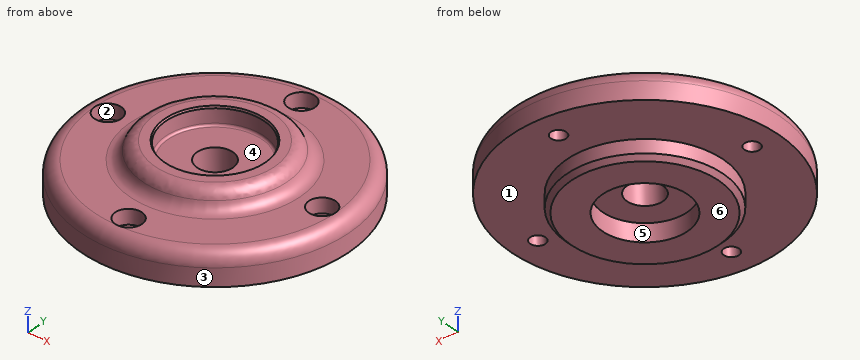
Autodesk Inventor part; units mm, degrees
ref_plane "YZ Plane" through (0, 0, 0) normal (1, 0, 0) x (0, 1, 0)
ref_plane "XZ Plane" through (0, 0, 0) normal (0, 1, 0) x (-1, 0, 0)
ref_plane "XY Plane" through (0, 0, 0) normal (0, 0, 1) x (1, 0, 0)
sketch "스케치4" plane through (0, 0, 0) normal (0, 0, 1) x (1, 0, 0)
  circle A0 centre (0, 0) radius 30
  dimension "d28" = 60
extrude "돌출4" add sketch "스케치4" along normal blind 7
sketch "스케치5" plane through (0, 0, 7) normal (0, 0, 1) x (1, 0, 0)
  circle A0 centre (0, 0) radius 16
  dimension "d31" = 32
extrude "돌출5" add sketch "스케치5" along normal blind 4
sketch "스케치6" plane through (0, 0, 0) normal (0, 0, -1) x (-1, 0, 0)
  circle A0 centre (0, 0) radius 17.5
  dimension "d34" = 35
extrude "돌출6" add sketch "스케치6" along normal blind 4
sketch "스케치8" plane through (0, 0, 11) normal (0, 0, 1) x (1, 0, 0)
  circle A0 centre (0, 0) radius 11
  dimension "d41" = 22
extrude "돌출8" cut sketch "스케치8" against normal blind 4
sketch "스케치9" plane through (0, 0, -4) normal (0, 0, -1) x (-1, 0, 0)
  circle A0 centre (0, 0) radius 9.5
  dimension "d44" = 19
extrude "돌출9" cut sketch "스케치9" against normal blind 4
sketch "스케치11" plane through (0, 0, 7) normal (0, 0, 1) x (1, 0, 0)
  circle A0 centre (0, 0) radius 4
  dimension "d49" = 8
extrude "돌출10" cut sketch "스케치11" against normal up to next
sketch "스케치12" plane through (0, 0, 7) normal (0, 0, 1) x (1, 0, 0)
  circle A0 centre (0, 24) radius 3
  point P0 (0, 0)
  dimension "d61" = 6
  dimension "d62" = 24
hole "구멍1" at (0, 24, 7) direction (0, 0, -1) diameter 3.4 end through all counterbore diameter 6 counterbore depth 3.3
pattern_circular "원형 패턴2" count 4 over 360 about axis through (0, 0, 7) along (0, 0, -1) of "구멍1"
fillet "모깎기3" radius 3 3 edges at (-30, 0, 7) (-16, 0, 7) (-16, 0, 11)
chamfer "모따기5" distance 1 angle 45 1 edges at (17.5, 0, -4)
chamfer "모따기6" distance 0.4 angle 30 1 edges at (-11, 0, 11) measured on face at (10.9643, -0.8851, 8.3333)
fillet "모깎기4" radius 0.5 1 edges at (-11, 0, 7)
properties part number "도면2-3번"
CAD build for the part. Positions are in the model's coordinates, mm. Face numbers are marked on the shaded views. A direction names the side the tool comes from. Round coordinates to 2 decimals unless told otherwise and drop trailing zeros. Order: outer loops, then holes, each group sorted by start corner. A loop starts at its lowest first (then second) coordinate and runs counter-clockwise, first axis right, second up.
Item 1: Tool access for the marked faces 4, 5 and 6: list every direction of +Z, -Z, +X, -X, +Y, -Y with a clear straight run to the whole face (end or side of a thin tool).
Item 2: Mould opens along Y. For the marked faces 1, 2 and 3 say: pulls with the +Y half, pulls with the -Y half, needs draft (parallel to the pull), parting line crosses it, or undercut.
Item 3: Pin check, flat tips, straight feed: pin 1 (7 mm diameter, centred on x = 0, y = 0, fed in from +Z); pin 2 (6.5 mm diameter, centred on x = 0, y = -24, fed in from +Z); pin 3 (6 mm diameter, centred on y = -15, z = 9.5, fed in from +X); pin 4 (8 mm diameter, centred on x = 24, y = 0, fed in from -Z). Stop position of each tip, or through.
Item 4: Saw through at C-C on z = 5.5. Write the cut outline in (x, y).
Item 5: Saw through at B-B on y = 0. State how many separate pieces and enclosed holes the cut face has, then the cut area to 3 significant figures.
Item 6: Probe line 1 along X through (y, z) = (-0.5, 5); line 2 along X through (y, z) = (24, 5.95); line 3 along X through (y, z) = (24, 0.95). List the from-to ranges inside material, lowest first.
Item 7: Saw through at A-A on z = 1. Write the cut outline in (x, y).
Reported:
1. face 4: +Z
1. face 5: -Z
1. face 6: -Z, +X, -X, +Y, -Y
2. face 1: needs draft
2. face 2: undercut
2. face 3: parting line crosses it
3. pin 1: passes through
3. pin 2: stops at z = 7
3. pin 3: stops at x = 24.69
3. pin 4: stops at z = 0
4. outline: circle Ø59.2 at (0, 0); hole circle Ø6 at (-24, 0); hole circle Ø8 at (0, 0); hole circle Ø6 at (0, -24); hole circle Ø6 at (0, 24); hole circle Ø6 at (24, 0)
5. separate pieces: 4
5. enclosed holes: 0
5. area: 400 mm2
6. line 1: x = -29.82 to -26.96, -21.04 to -3.97, 3.97 to 21.04, 26.96 to 29.82
6. line 2: x = -16.77 to -3, 3 to 16.77
6. line 3: x = -18 to -1.7, 1.7 to 18
7. outline: circle Ø60 at (0, 0); hole circle Ø3.4 at (-24, 0); hole circle Ø8 at (0, 0); hole circle Ø3.4 at (0, -24); hole circle Ø3.4 at (0, 24); hole circle Ø3.4 at (24, 0)
